Study the drawing (mm; zero at the part's minimum x, y, z) and answer. A direction names the side the tool comes from. Round coordinates to 2 decimals unless told otherwise and drop trailing zeros. Write each loop counter-clockwise with the first axis right and the second up, starting at its lowest first coordinate (ties: lowest second). Pieces come first, ordered by that corner, then holes.
(1) Each of these flat-tipped pins is pushed along its axis until it touches: pin 1 Ø3 at (y, z) = (81, 46) entering from -X; pin 2 Ø6 at (x, y) = (38.5, 66.5) entering from +Z; pin 3 Ø1 at (x, z) = (82.5, 12) entering from +Y; pin 4 Ø2 at (x, z) = (53.5, 84) entering from -Y. Where does it stop, or does it pass through?
(2) A cutting plane is placed at A-A, the plane x = 36. Give the vertices of the cut face in (y, z), and give its area (3 significant figures).
(3) A cutting plane is placed at C-C, the plane z = 15. Give the vertices of the cut face in (x, y), and give its area (3 significant figures).
(4) A cutting plane is placed at B-B, the plane y = 30. Give the vertices of the cut face in (x, z).
(5) Find the intervals of material crossed by probe 1 along Y at (x, z) = (93, 61); probe 2 along Z at (x, y) = (90.5, 18.5); probe 3 along X at (y, z) = (18.5, 85), in increasing order.
(6) For the marked faces 1 and 2, determine the directions among +Z, -Z, +X, -X, +Y, -Y from which every point of the face is accessible in a straight line to the end or side of a thin tool.
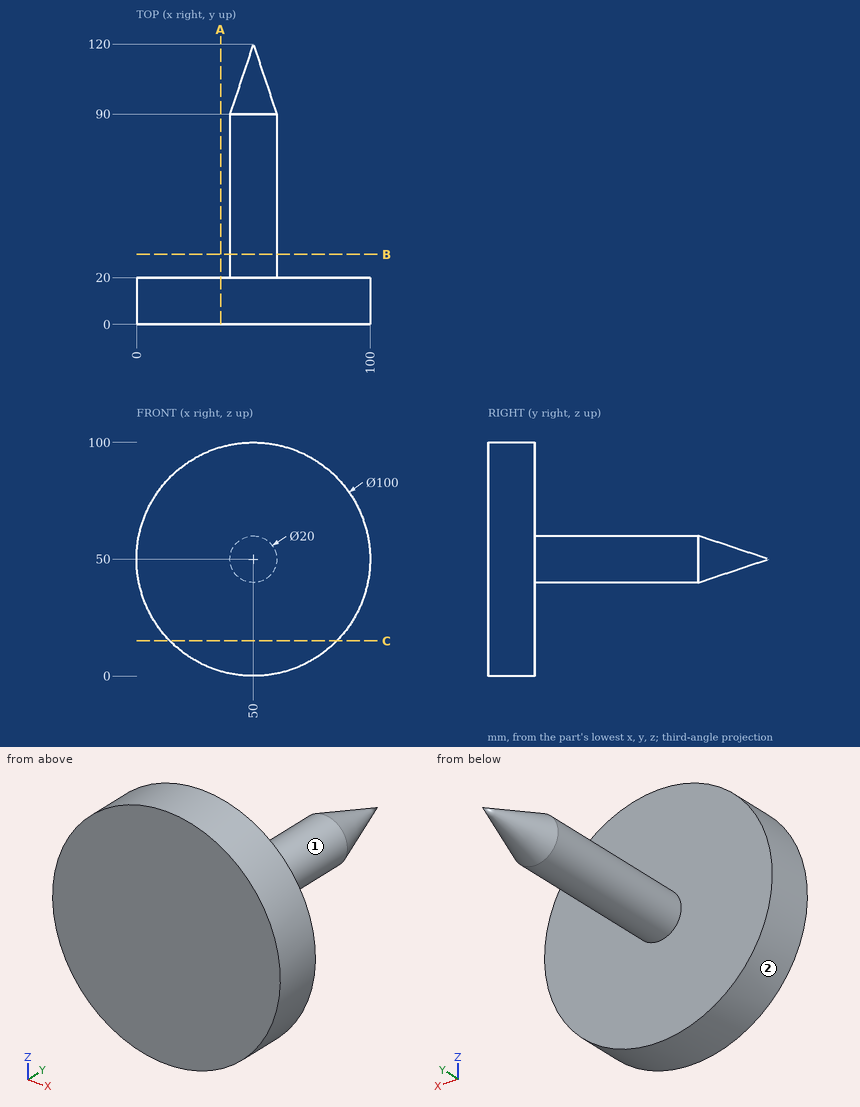
Solutions:
1. pin 1: stops at x = 40.32
1. pin 2: stops at z = 55.27
1. pin 3: stops at y = 20
1. pin 4: stops at y = 0
2. outline: (0, 2) - (20, 2) - (20, 98) - (0, 98) - close
2. area: 1,920 mm2
3. outline: (14.29, 0) - (85.71, 0) - (85.71, 20) - (14.29, 20) - close
3. area: 1,430 mm2
4. outline: circle Ø20 at (50, 50)
5. probe 1: y = 0 to 20
5. probe 2: z = 20.68 to 79.32
5. probe 3: x = 14.29 to 85.71
6. face 1: +Y
6. face 2: +Y, -Y
